```python
from build123d import *

# Parameters (mm, degrees)
F2_R      = 0.75
F10_R     = 0.25
F15_R     = 0.75
F19_DEPTH = 0.75


# Not quite as in the source:
# - a feature of the source that left no trace in its solid (it failed there, or was rolled back) is left out
# - a pattern or mirror of a feature is missing from the dataset's text; its kind, count and spacing are read off the source's solid


with BuildPart() as f3:
    # F3: sweep along a path in F0
    with BuildLine(Plane.XZ) as f3_path:
        Line((-30, 0), (0, 0))
        Line((0, 0), (30, 0))
    # F2 (on plane+point) → F3 (sweep)
    with BuildSketch(Plane.YZ.offset(-30)):
        Circle(F2_R)
    sweep(path=f3_path.line)

    # F11: sweep along a path in F8
    with BuildLine(Plane.XZ) as f11_path:
        Line((0, 0), (33.02, 0))
    # F10 (on plane+point) → F11 (sweep)
    with BuildSketch(Plane.YZ.offset(33.02)):
        Circle(F10_R)
    f11 = sweep(path=f11_path.line)

    # F11_copies: F11 across plane
    add(f11.mirror(Plane(origin=(-0.001764, 0, 0), x_dir=(0, 0, -1), z_dir=(-1, 0, 0))))

    # F16: sweep along a path in F13
    with BuildLine(Plane.YZ) as f16_path:
        Line((0, 0), (-50, 0))
    # F15 (on plane+point) → F16 (sweep)
    with BuildSketch(Plane.XZ.offset(50)):
        Circle(F15_R)
    sweep(path=f16_path.line)

    # F18 (on plane+point) → F19 (join, symmetric)
    with BuildSketch(Plane.YZ):
        Polygon((-50, -1.4374784192), (-50, 0), (-50, 2.8882389888), (-56.6018782556, 2.8882389888), (-56.6018782556, 1.3868947281), (-52.8817437589, 1.3868947281), (-52.8817437589, 0), (-59.6723221242, 0), (-59.6723221242, -1.4374784192), align=None)
    extrude(amount=F19_DEPTH, both=True)


solid = f3.part
```
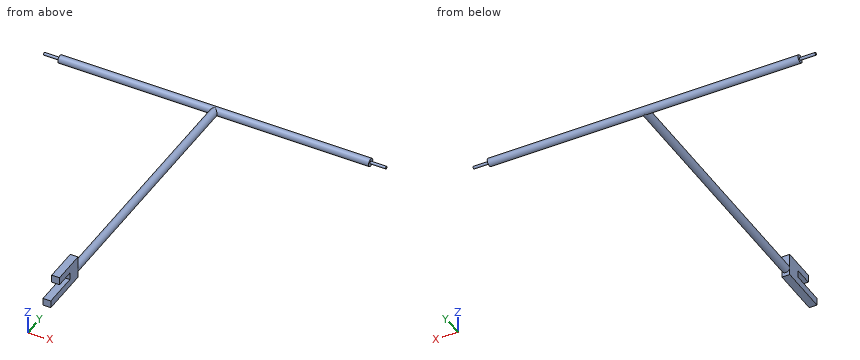
The listing builds one solid part. Answer for the finished solid, in the listing's coordinates (mm). Give positions to 0.01 mm unless a question says otherwise; leave off trailing zeros. Order: outer loops, then holes, each group sorted by start corner. A loop starts at its lowest first (then second) coordinate and runs counter-clockwise, first axis right, second up. Notation, with made-up numbers: (46.25, 15.25) -> (52.25, 15.25) arc R21 cw to (52.25, 48.25) -> close; hole circle Ø6 at (7.25, -26). An arc over 180 degrees is marked (long way). Answer as a JSON object with one key per item and string values. Group by question number.
Item 1: Consider L1, parallel to Y at x = 28, z = -0.15; L2, parallel to Y at x = -3.5, z = -0.4; L3, parallel to X at y = -26, z = -0.3. Determine where each line is inside the solid, lowest interval first. Write a range as from..to.
Item 2: The part is cut by section A-A on x = 0. Write down the section's boundary in (y, z).
Item 3: Flat-ended cylindrical pins translate along their axes: pin 1 (5 mm diameter, centred on x = 5.5, y = -6, fed in from -Z); pin 2 (1 mm diameter, centred on y = -14, z = -0.5, fed in from +X); pin 3 (4 mm diameter, centred on x = 1, y = -6.5, fed in from -Z); pin 4 (0.7 mm diameter, centred on x = 0, z = -0.5, fed in from +Y). Find the tip coordinate at first contact, or state that the pin passes through.
Item 4: The part is cut by section B-B on y = -14.5. Write down the section's boundary in (x, z), and give its area (3 significant figures).
Result set:
{
 "1": {"L1": "-0.73..0.73", "L2": "-0.63..0.63", "L3": "-0.69..0.69"},
 "2": {"outline": "(-59.67, -1.44) -> (-50, -1.44) -> (-50, -0.75) -> (0, -0.75) arc R0.75 ccw to (0, 0.75) -> (-50, 0.75) -> (-50, 2.89) -> (-56.6, 2.89) -> (-56.6, 1.39) -> (-52.88, 1.39) -> (-52.88, 0) -> (-59.67, 0) -> close"},
 "3": {"pin 1": "through", "pin 2": "x = 0.75", "pin 3": "z = -0.75", "pin 4": "y = 0.73"},
 "4": {"outline": "circle Ø1.5 at (0, 0)", "area": "1.77 mm²"}
}
